Input: part model. Units: mm. Frame: model coordinates. A direction names the side the tool comes from. Coordinates: 2 decimals unless noted, no trailing zeros. Write each loop counter-clockwise with the first axis right and the second up, starting at its lowest first coordinate (ties: lowest second). Pieces come first, ordered by that corner, then holes. Notation, with made-up numbers: (24.5, 69) - (49.5, 69) arc R24 ccw to (49.5, 89) - close; hole circle Ø10 at (76.5, 59). An arc over 180 degrees is marked (long way). Put each result on its own line as item: value. Start each with the question number.
1. Cut plane B-B, the plane x = 0. Return loops of the section in (y, z), and give its area (3 significant figures).
2. Pull-direction query (Y, two-part tool) for faces 1 (the flat face through (-1, 72, 30)), 2 (the flat face through (-1, -72, 16)), 3 (the flat face through (-1, 1, 2)), 4 (the flat face through (-41, -1, 30)); classes: released by +Y, released by -Y, zero draft, split by the parting line, or undercut.
3. Cut plane C-C, the plane y = -56. Return loops of the section in (x, z), and give its area (3 significant figures).
4. Cut plane D-D, the plane z = 52.5. Return loops of the section in (x, y), and give its area (3 significant figures).
5. Access query for faces 5 (the flat face through (39, -1, 31)), 6 (the cylindrical face through (0.79, -70.99, 24.01)), 7 (the flat face through (-40, 0, 60)). Directions: +Z, -Z, +X, -X, +Y, -Y. A direction counts if a zero-diameter tool reaches every point of the face in a straight line with its end or side. Return the directions, or none.
6. Line query: line 1 (X direction, y = -20.5, z = 52.5); line 2 (Y direction, x = -36, z = 36); line 3 (Z direction, x = -23, y = -17). Output: solid intervals per line, ascending.
7. Cut plane A-A, the plane z = 21.5. Return loops of the section in (x, y).
8. Pin query (flat end, axial travel): pin 1 (12 mm diameter, centred on x = 28.5, y = -43.5, fed in from +Z); pin 2 (10 mm diameter, centred on x = 1.5, z = 49, fed in from -Y). Return the tip coordinate at first contact, or that it passes through.
from build123d import *

# Parameters (mm, degrees)
F0_W     = 78
F0_H     = 140
F1_DEPTH = 2
F0_W_2   = 82
F0_H_2   = 144
F2_DEPTH = 60
F4_DEPTH = 25
F5_R     = 2


# Not quite as in the source:
# - a feature names something its author has since deleted; it is built from what else it names


with BuildPart() as f1:
    # F0 (on Top) → F1 (new body)
    with BuildSketch(Plane.XY):
        Rectangle(F0_W, F0_H)
    extrude(amount=F1_DEPTH)

    # F0 (on Top) → F2 (join)
    with BuildSketch(Plane.XY):
        Rectangle(F0_W_2, F0_H_2)
        Rectangle(F0_W, F0_H, mode=Mode.SUBTRACT)
    extrude(amount=F2_DEPTH)

    # F3 (on face) → F4 (cut)
    with BuildSketch(Plane(origin=(0, -70, 0), x_dir=(-1, 0, 0), z_dir=(0, 1, 0))):
        with BuildLine():
            Line((36, 60), (-36, 60))
            ThreePointArc((-36, 60), (0, 24), (36, 60))
        make_face()
    extrude(amount=-F4_DEPTH, mode=Mode.SUBTRACT)

    # F5
    f5_edges = [f1.edges().sort_by_distance(p)[0] for p in [
        (-41, 72, 30),
        (41, 72, 30),
        (-41, -72, 30),
        (41, -72, 30),
    ]]
    fillet(f5_edges, radius=F5_R)


solid = f1.part
Report:
1. outline: (-72, 0) - (72, 0) - (72, 60) - (70, 60) - (70, 2) - (-70, 2) - (-70, 24) - (-72, 24) - close
1. area: 448 mm^2
2. face 1: released by +Y
2. face 2: released by -Y
2. face 3: undercut
2. face 4: zero draft
3. outline: (-41, 0) - (41, 0) - (41, 60) - (39, 60) - (39, 2) - (-39, 2) - (-39, 60) - (-41, 60) - close
3. area: 396 mm^2
4. outline: (-41, -70) arc R2 ccw to (-39, -72) - (-35.21, -72) - (-35.21, -70) - (-39, -70) - (-39, 70) - (39, 70) - (39, -70) - (35.21, -70) - (35.21, -72) - (39, -72) arc R2 ccw to (41, -70) - (41, 70) arc R2 ccw to (39, 72) - (-39, 72) arc R2 ccw to (-41, 70) - close
4. area: 744 mm^2
5. face 5: +Z
5. face 6: +Z, -Y
5. face 7: +Z, +X, -X, +Y, -Y
6. line 1: x = -41 to -39, 39 to 41
6. line 2: y = -72 to -70, 70 to 72
6. line 3: z = 0 to 2
7. outline: (-41, -70) arc R2 ccw to (-39, -72) - (39, -72) arc R2 ccw to (41, -70) - (41, 70) arc R2 ccw to (39, 72) - (-39, 72) arc R2 ccw to (-41, 70) - close; hole (-39, -70) - (39, -70) - (39, 70) - (-39, 70) - close
8. pin 1: stops at z = 2
8. pin 2: stops at y = 70
